Design review of the part built by this model. Coordinates are the model's own, in mm. Give positions to 0.01 mm unless a question says otherwise; leave off trailing zeros. Loops run counter-clockwise (first coordinate to the right, second up) from the corner with the lowest first, then second, coordinate; pieces in that order, holes last. Notation, with made-up numbers: M 23,44 L 76,44 A30 cw 76,79 Z; hole C 30.5,78.25 d6. An arc over 180 degrees is marked long. Use CSV: the item, a comma, the result in double quotes.
from build123d import *

# Parameters (mm, degrees)
SKETCH_1_W              = 337.35
SKETCH_1_H              = 116.87
SKETCH_1_W_2            = 324.05
SKETCH_1_H_2            = 103.07
EXTRUDE_1_DEPTH         = 8
FILLET_1_R              = 5
HOLE_WIZARD_3_2_3_2_1_D = 3.2
SKETCH_5_W              = 32
SKETCH_5_H              = 1.5
CUT_EXTRUDE_1_DEPTH     = 355.911853
EXTRUDE_2_REACH         = 356.912
SKETCH_6_W              = 3
SKETCH_6_H              = 8
SKETCH_7_W              = 257.05
SKETCH_7_H              = 8
EXTRUDE_3_DEPTH         = 4
SKETCH_8_W              = 257.05
SKETCH_8_H              = 4
EXTRUDE_4_DEPTH         = 3
SKETCH_11_W             = 99.07
SKETCH_11_H             = 11
EXTRUDE_5_DEPTH         = 2
SKETCH_13_W             = 42
SKETCH_13_H             = 4.5
CUT_EXTRUDE_2_DEPTH     = 354.692894189
SKETCH_14_W             = 121.5
SKETCH_14_H             = 1.5
CUT_EXTRUDE_3_DEPTH     = 355.911853
SKETCH_16_W             = 32
SKETCH_16_H             = 6.5
EXTRUDE_7_DEPTH         = 4
SKETCH_17_W             = 103.07
SKETCH_17_H             = 3
CUT_EXTRUDE_4_DEPTH     = 0.1
EXTRUDE_8_DEPTH         = 2
SKETCH_19_W             = 70.55
SKETCH_19_H             = 2
SKETCH_19_W_2           = 95
EXTRUDE_9_DEPTH         = 3
SKETCH_20_R             = 3.5
CUT_EXTRUDE_5_DEPTH     = 4
SKETCH_21_R             = 3.1
CUT_EXTRUDE_6_DEPTH     = 2
EXTRUDE_10_DEPTH        = 2
EXTRUDE_10_DEPTH_BACK   = 3
SKETCH_22_W             = 6
SKETCH_22_H             = 6
SKETCH_22_R             = 1.5
SKETCH_23_W             = 10
SKETCH_23_H             = 1.5
SKETCH_23_W_2           = 15
CUT_EXTRUDE_7_DEPTH     = 6.9
SKETCH_24_W             = 103.07
SKETCH_24_H             = 3
CUT_EXTRUDE_8_DEPTH     = 358.110094229
SKETCH_25_W             = 402.768513644
SKETCH_25_H             = 192.082702388
SKETCH_25_W_2           = 190
SKETCH_25_H_2           = 48.964424343
CUT_EXTRUDE_9_DEPTH     = 358.110094229
CHAMFER_1_SIZE          = 5


with BuildPart() as part:
    # 草图1 → 凸台-拉伸1 (new body)
    with BuildSketch(Plane(origin=(0, 0, 0), x_dir=(1, 0, 0), z_dir=(0, 1, 0))):
        with Locations((168.675, 58.435)):
            Rectangle(SKETCH_1_W, SKETCH_1_H)
        with Locations((168.925, 58.435)):
            Rectangle(SKETCH_1_W_2, SKETCH_1_H_2, mode=Mode.SUBTRACT)
    extrude(amount=EXTRUDE_1_DEPTH)

    # 圆角1
    fillet_1_edges = [part.edges().sort_by_distance(p)[0] for p in [
        (0, 4, -116.87),
        (337.35, 4, -116.87),
        (337.35, 4, 0),
        (0, 4, 0),
    ]]
    fillet(fillet_1_edges, radius=FILLET_1_R)

    # Ø3.2 (3.2) 直径孔1 (through all)
    with Locations(Plane(origin=(0, 8, 0), x_dir=(1, 0, 0), z_dir=(0, 1, 0))):
        with Locations((3.45, 98.435), (87.17, 113.42), (247.17, 113.42), (334.15, 98.435), (334.15, 18.435), (247.17, 3.45), (87.17, 3.45), (3.45, 18.435)):
            Hole(HOLE_WIZARD_3_2_3_2_1_D / 2)

    # 草图5 → 切除-拉伸1 (cut, through all)
    with BuildSketch(Plane.XY.offset(-109.97)):
        with Locations((57.9, 0.75)):
            Rectangle(SKETCH_5_W, SKETCH_5_H)
    extrude(amount=-CUT_EXTRUDE_1_DEPTH, mode=Mode.SUBTRACT)

    # 草图6 → 凸台-拉伸2 (add, up to next)
    with BuildSketch(Plane.XY.offset(-109.97), mode=Mode.PRIVATE) as extrude_2_sk1:
        with Locations((40.4, 4)):
            Rectangle(SKETCH_6_W, SKETCH_6_H)
    extrude_2_tool1 = extrude(extrude_2_sk1.sketch, amount=EXTRUDE_2_REACH, mode=Mode.PRIVATE) - part.part
    add(extrude_2_tool1.solids().sort_by_distance((40.4, 4, -109.97))[0])

    # 草图7 → 凸台-拉伸3 (add)
    with BuildSketch(Plane.XY.offset(-109.97)):
        with Locations((202.425, 4)):
            Rectangle(SKETCH_7_W, SKETCH_7_H)
    extrude(amount=EXTRUDE_3_DEPTH)

    # 草图8 → 凸台-拉伸4 (add)
    with BuildSketch(Plane.XZ):
        with Locations((202.425, -107.97)):
            Rectangle(SKETCH_8_W, SKETCH_8_H)
    extrude(amount=EXTRUDE_4_DEPTH)

    # 草图11 → 凸台-拉伸5 (add)
    with BuildSketch(Plane.ZY.offset(-330.95)):
        with Locations((-56.435, 2.5)):
            Rectangle(SKETCH_11_W, SKETCH_11_H)
    extrude(amount=EXTRUDE_5_DEPTH)

    # 草图13 → 切除-拉伸2 (cut, through all)
    with BuildSketch(Plane.XY.offset(-105.97)):
        with Locations((307.95, -0.75)):
            Rectangle(SKETCH_13_W, SKETCH_13_H)
    extrude(amount=-CUT_EXTRUDE_2_DEPTH, mode=Mode.SUBTRACT)

    # 草图14 → 切除-拉伸3 (cut, through all)
    with BuildSketch(Plane(origin=(0, 0, -6.9), x_dir=(-1, 0, 0), z_dir=(0, 0, -1))):
        with Locations((-173.2, 0.75)):
            Rectangle(SKETCH_14_W, SKETCH_14_H)
    extrude(amount=-CUT_EXTRUDE_3_DEPTH, mode=Mode.SUBTRACT)

    # 草图16 → 凸台-拉伸7 (add)
    with BuildSketch(Plane.XY.offset(-109.97)):
        with Locations((57.9, 4.75)):
            Rectangle(SKETCH_16_W, SKETCH_16_H)
    extrude(amount=EXTRUDE_7_DEPTH)

    # 草图17 → 切除-拉伸4 (cut)
    with BuildSketch(Plane(origin=(330.95, 0, 0), x_dir=(0, 0, -1), z_dir=(1, 0, 0))):
        with Locations((58.435, -1.5)):
            Rectangle(SKETCH_17_W, SKETCH_17_H)
    extrude(amount=-CUT_EXTRUDE_4_DEPTH, mode=Mode.SUBTRACT)

    # 草图18 → 凸台-拉伸8 (add)
    with BuildSketch(Plane(origin=(0, 0, -6.9), x_dir=(-1, 0, 0), z_dir=(0, 0, -1))):
        Polygon((-233.95, 0), (-233.95, 1.5), (-112.45, 1.5), (-112.45, 0), (-41.9, 0), (-41.9, 8), (-328.95, 8), (-328.95, 0), align=None)
    extrude(amount=EXTRUDE_8_DEPTH)

    # 草图19 → 凸台-拉伸9 (add)
    with BuildSketch(Plane.XZ):
        with Locations((77.175, -7.9)):
            Rectangle(SKETCH_19_W, SKETCH_19_H)
        with Locations((281.45, -7.9)):
            Rectangle(SKETCH_19_W_2, SKETCH_19_H)
    extrude(amount=EXTRUDE_9_DEPTH)

    # 草图20 → 切除-拉伸5 (cut)
    with BuildSketch(Plane.XZ.offset(3)):
        with Locations((92.088456012, -9.54)):
            Circle(SKETCH_20_R)
        with Locations((262.268456012, -9.54)):
            Circle(SKETCH_20_R)
        with Locations((328.308456012, -13.35)):
            Circle(SKETCH_20_R)
        with Locations((328.308456012, -74.31)):
            Circle(SKETCH_20_R)
        with Locations((137.808456012, -107.33)):
            Circle(SKETCH_20_R)
        with Locations((22.238456012, -9.54)):
            Circle(SKETCH_20_R)
        with Locations((9.538456012, -23.51)):
            Circle(SKETCH_20_R)
        with Locations((9.538456012, -103.52)):
            Circle(SKETCH_20_R)
    extrude(amount=-CUT_EXTRUDE_5_DEPTH, mode=Mode.SUBTRACT)

    # 草图21 → 切除-拉伸6 (cut)
    with BuildSketch(Plane(origin=(0, 8, 0), x_dir=(1, 0, 0), z_dir=(0, 1, 0))):
        with Locations(Location((87.17, 113.42, 0), (0, 0, 270))):
            Circle(SKETCH_21_R)
        with Locations(Location((247.17, 113.42, 0), (0, 0, 270))):
            Circle(SKETCH_21_R)
        with Locations(Location((334.15, 98.435, 0), (0, 0, 270))):
            Circle(SKETCH_21_R)
        with Locations(Location((334.15, 18.435, 0), (0, 0, 270))):
            Circle(SKETCH_21_R)
        with Locations(Location((247.17, 3.45, 0), (0, 0, 270))):
            Circle(SKETCH_21_R)
        with Locations(Location((87.17, 3.45, 0), (0, 0, 270))):
            Circle(SKETCH_21_R)
        with Locations(Location((3.45, 18.435, 0), (0, 0, 270))):
            Circle(SKETCH_21_R)
        with Locations(Location((3.45, 98.435, 0), (0, 0, 270))):
            Circle(SKETCH_21_R)
    extrude(amount=-CUT_EXTRUDE_6_DEPTH, mode=Mode.SUBTRACT)

    # 草图22 → 凸台-拉伸10 (add, two sides: drawn at the far end of the back side and taken through both)
    # profile 1 of 4: a face of its own
    with BuildSketch(Plane(origin=(0, 4, 0), x_dir=(1, 0, 0), z_dir=(0, 1, 0)).offset(-EXTRUDE_10_DEPTH_BACK)):
        with Locations((9.9, 106.97)):
            Rectangle(SKETCH_22_W, SKETCH_22_H)
        with Locations(Location((9.9, 106.97, 0), (0, 0, 90))):
            Circle(SKETCH_22_R, mode=Mode.SUBTRACT)
    # profile 2 of 4: a face of its own
    with BuildSketch(Plane(origin=(0, 4, 0), x_dir=(1, 0, 0), z_dir=(0, 1, 0)).offset(-EXTRUDE_10_DEPTH_BACK)):
        with Locations((35.9, 106.97)):
            Rectangle(SKETCH_22_W, SKETCH_22_H)
        with Locations(Location((35.9, 106.97, 0), (0, 0, 90))):
            Circle(SKETCH_22_R, mode=Mode.SUBTRACT)
    # profile 3 of 4: a face of its own
    with BuildSketch(Plane(origin=(0, 4, 0), x_dir=(1, 0, 0), z_dir=(0, 1, 0)).offset(-EXTRUDE_10_DEPTH_BACK)):
        with Locations((9.9, 9.9)):
            Rectangle(SKETCH_22_W, SKETCH_22_H)
        with Locations(Location((9.9, 9.9, 0), (0, 0, 90))):
            Circle(SKETCH_22_R, mode=Mode.SUBTRACT)
    # profile 4 of 4: a face of its own
    with BuildSketch(Plane(origin=(0, 4, 0), x_dir=(1, 0, 0), z_dir=(0, 1, 0)).offset(-EXTRUDE_10_DEPTH_BACK)):
        with Locations((35.9, 9.9)):
            Rectangle(SKETCH_22_W, SKETCH_22_H)
        with Locations(Location((35.9, 9.9, 0), (0, 0, 90))):
            Circle(SKETCH_22_R, mode=Mode.SUBTRACT)
    extrude(amount=EXTRUDE_10_DEPTH + EXTRUDE_10_DEPTH_BACK)

    # 草图23 → 切除-拉伸7 (cut)
    with BuildSketch(Plane.ZY):
        with Locations((-63.435, 0.75)):
            Rectangle(SKETCH_23_W, SKETCH_23_H)
        with Locations((-50.935, 0.75)):
            Rectangle(SKETCH_23_W_2, SKETCH_23_H)
    extrude(amount=-CUT_EXTRUDE_7_DEPTH, mode=Mode.SUBTRACT)

    # 草图24 → 切除-拉伸8 (cut, through all)
    with BuildSketch(Plane(origin=(337.35, 0, 0), x_dir=(0, 0, -1), z_dir=(1, 0, 0))):
        with Locations((58.435, -1.5)):
            Rectangle(SKETCH_24_W, SKETCH_24_H)
    extrude(amount=-CUT_EXTRUDE_8_DEPTH, mode=Mode.SUBTRACT)

    # 草图25 → 切除-拉伸9 (cut, through all)
    with BuildSketch(Plane(origin=(0, 8, 0), x_dir=(1, 0, 0), z_dir=(0, 1, 0))):
        with Locations((167.276381716, 50.966242561)):
            Rectangle(SKETCH_25_W, SKETCH_25_H)
        with Locations((167.17, 6.206921893)):
            Rectangle(SKETCH_25_W_2, SKETCH_25_H_2, mode=Mode.SUBTRACT)
    extrude(amount=-CUT_EXTRUDE_9_DEPTH, mode=Mode.SUBTRACT)

    # 倒角1
    chamfer_1_edges = [part.edges().sort_by_distance(p)[0] for p in [
        (72.17, 8, -4.45),
        (262.17, 8, -4.45),
    ]]
    chamfer(chamfer_1_edges, length=CHAMFER_1_SIZE)


solid = part.part
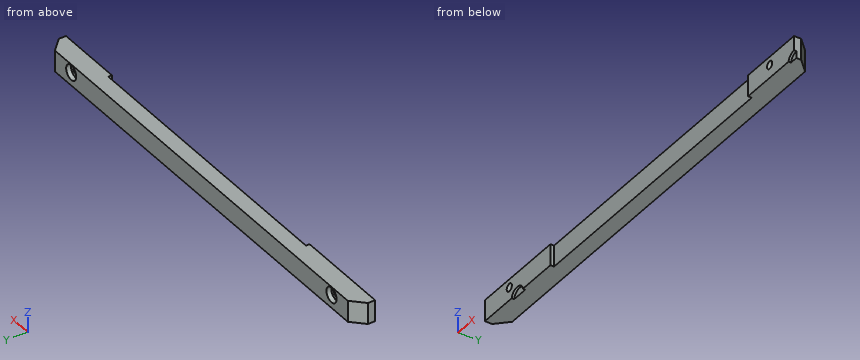
(1) Clearance check with flat-ended pins moving along their axes: P1, Ø4, axis at x = 152, z = -7.5, coming from the -Y side; P2, Ø2, axis at y = 4.5, z = -7, coming from the +X side; P3, Ø1.9, axis at x = 247.17, z = -3.45, coming from the +Y side; P4, Ø1, axis at y = 6, z = -5, coming from the +X side. State where each tip first meets the part, or that it passes through.
A:
P1,"y = 1.5"
P2,"x = 261.67"
P3,"through"
P4,"x = 259.67"
(2) We need section B-B on z = -3.45. State the section outline as (x, y) points.
A:
outline,"M 72.17,0 L 85.57,0 L 85.57,6 L 84.07,6 L 84.07,8 L 77.17,8 L 72.17,3 Z; M 88.77,0 L 112.45,0 L 112.45,1.5 L 233.95,1.5 L 233.95,0 L 245.57,0 L 245.57,6 L 244.07,6 L 244.07,8 L 90.27,8 L 90.27,6 L 88.77,6 Z; M 248.77,0 L 262.17,0 L 262.17,3 L 257.17,8 L 250.27,8 L 250.27,6 L 248.77,6 Z"
(3) We need section C-C on x = 202. State the section outline as (y, z) points.
A:
outline,"M 1.5,-8.9 L 8,-8.9 L 8,0 L 1.5,0 Z"
(4) Wall thickness on line 1 along Z through (x, y) = (247.17, 4.6); line 2 along X through (y, z) = (4, -3.75); line 3 along X through (y, z) = (5.75, -3.5): over which ranges is each line inside the solid? List them lowest first. Write a range as [from, to].
A:
line 1,"[-8.9, -5.05], [-1.85, 0]"
line 2,"[73.17, 85.6], [88.74, 245.6], [248.74, 261.17]"
line 3,"[74.92, 85.57], [88.77, 245.57], [248.77, 259.42]"
(5) We need section A-A on x = 247.17. State the section outline as (y, z) points, then the cut area to 3 significant figures.
A:
outline,"M 0,-8.9 L 8,-8.9 L 8,-6.55 L 6,-6.55 L 6,-5.05 L 0,-5.05 Z; M 0,-1.85 L 6,-1.85 L 6,-0.35 L 8,-0.35 L 8,0 L 0,0 Z"
area,"39.6 mm²"
